Geometry: see drawing. Coordinates: mm, zero at the bounding-box minimum. A direction names the side the tool comes from. Round coordinates to 2 decimals unless told otherwise and drop trailing zeros. Write each loop counter-clockwise with the first axis right and the second up, starting at its lowest first coordinate (ties: lowest second). Pieces come first, ordered by that corner, then holes. Notation, with made-up numbers: (63.25, -21.5) - (115.25, -21.5) arc R16 cw to (115.25, 2.5) - close; hole circle Ø5 at (74, 17.5). An arc over 180 degrees is marked (long way). Use a Markdown table: item, result. Add a question column.
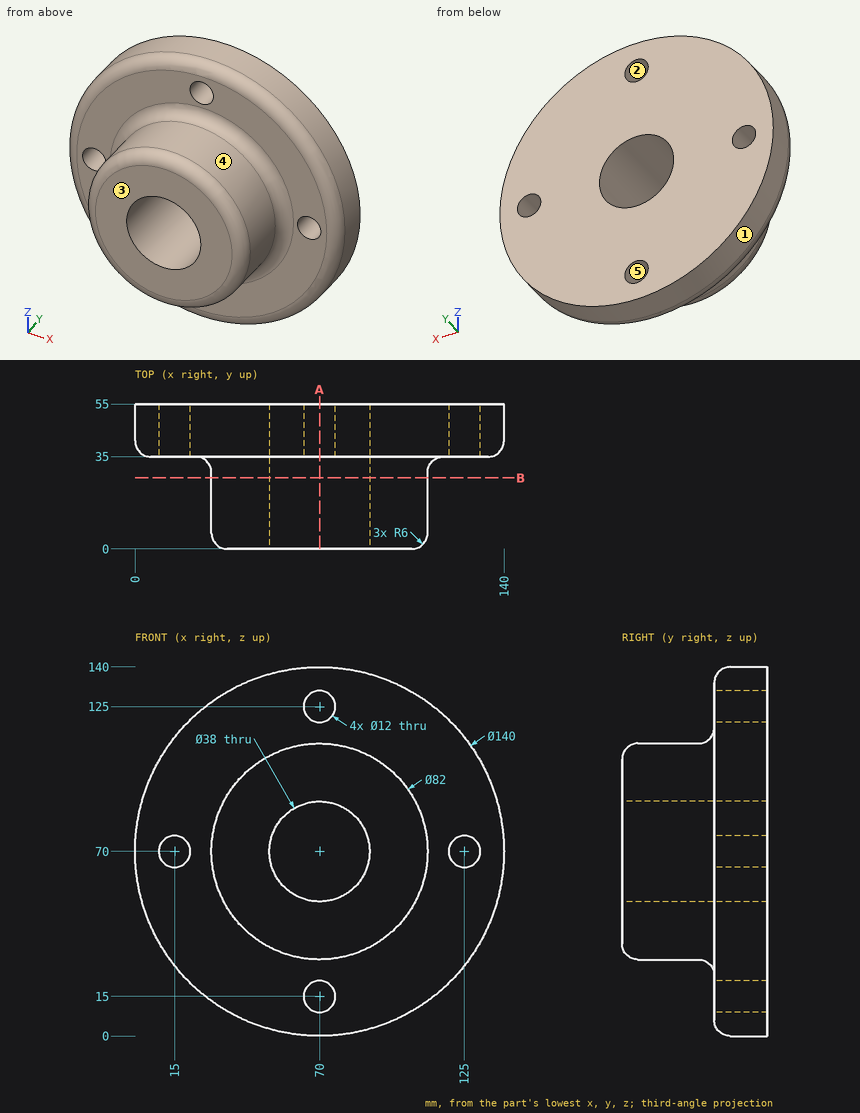
1) Set-up query: the marked faces 4 and 5. Return all of +Z, -Z, +X, -X, +Y, -Y with unobstructed straight access to the full face (end or side cutting, diameter ignored); none if empty.
2) Section A-A, the plane x = 70. Return the cut outline in (y, z), then the cut area to 3 significant figures.
3) Draft query along Z for the marked faces 1, 2 and 3. Return one class per face: released by +Z, released by -Z, zero draft, split by the parting line, or undercut.
4) Material intervals for L1, parallel to Z at x = 70, y = 45.5; L2, parallel to X at y = 43.5, z = 67.5; L3, parallel to X at y = 25, z = 70, sorted ascending. Write a range as from..to.
5) Section B-B, the plane y = 27. Return the cut outline in (x, z).
6) Pin query (flat end, axial travel): P1, Ø8, axis at x = 91.5, z = 14.5, coming from the -Y side; P2, Ø19, axis at x = 70, z = 125, coming from the -Y side; P3, Ø3, axis at x = 29.5, y = 37, coming from the +Z side. Return the tip coordinate at first contact, or that it passes through.
Output values:
| question | item | result |
|---|---|---|
| 1 | face 4 | -Y |
| 1 | face 5 | +Y, -Y |
| 2 | outline | (0, 35) arc R6 ccw to (6, 29) - (29, 29) arc R6 cw to (35, 23) - (35, 21) - (55, 21) - (55, 51) - (0, 51) - close; (0, 89) - (55, 89) - (55, 119) - (35, 119) - (35, 117) arc R6 cw to (29, 111) - (6, 111) arc R6 ccw to (0, 105) - close; (35, 6) arc R6 ccw to (41, 0) - (55, 0) - (55, 9) - (35, 9) - close; (35, 131) - (55, 131) - (55, 140) - (41, 140) arc R6 ccw to (35, 134) - close |
| 2 | area | 3,080 mm^2 |
| 3 | face 1 | split by the parting line |
| 3 | face 2 | undercut |
| 3 | face 3 | zero draft |
| 4 | L1 | z = 0..9, 21..51, 89..119, 131..140 |
| 4 | L2 | x = 0.04..9.55, 20.45..51.17, 88.83..119.55, 130.45..139.96 |
| 4 | L3 | x = 29..51, 89..111 |
| 5 | outline | circle Ø82 at (70, 70); hole circle Ø38 at (70, 70) |
| 6 | P1 | stops at y = 35 |
| 6 | P2 | stops at y = 34.81 |
| 6 | P3 | stops at z = 126.9 |
